Geometry check sheet. Reference: the model listing, model coordinates, mm. A direction names the side the tool comes from. Round coordinates to 2 decimals unless told otherwise and drop trailing zeros. Write each loop counter-clockwise with the first axis right and the second up, starting at its lowest first coordinate (ties: lowest second). Pieces come first, ordered by that corner, then holes.
from build123d import *

# Parameters (mm, degrees)
F0_W     = 10
F0_H     = 10
F1_DEPTH = 2
F2_W     = 2
F2_H     = 10
F3_DEPTH = 8
F5_DEPTH = 50


with BuildPart() as f1:
    # F0 (on Top) → F1 (new body)
    with BuildSketch(Plane.XY):
        Rectangle(F0_W, F0_H)
    extrude(amount=F1_DEPTH)

    # F2 (on face) → F3 (join)
    with BuildSketch(Plane.XY.offset(2)):
        with Locations((-4, 0)):
            Rectangle(F2_W, F2_H)
        with Locations((4, 0)):
            Rectangle(F2_W, F2_H)
    extrude(amount=F3_DEPTH)

    # F4 (on face) → F5 (join)
    with BuildSketch(Plane(origin=(0, 5, 0), x_dir=(-1, 0, 0), z_dir=(0, 1, 0))):
        Polygon((-3, 10), (-5, 10), (-5, 0), (5, 0), (5, 10), (3, 10), (3, 2), (-3, 2), align=None)
    extrude(amount=F5_DEPTH)


solid = f1.part
1. Section check B-B (y = 9). Record the cut outline in (x, z), plus the area to 3 significant figures.
2. Section check A-A (z = 6.25). Record the cut outline in (x, y).
3. Depth check by flat-ended pin: pin 1 Ø3 at (x, y) = (0, 33.5) entering from +Z. Enter the tip coordinate at first touch or a pass-through.
4. Access from +Z, -Z, +X, -X, +Y, -Y to the whole of each face (thin tool, end or side, straight path). Record for faces 1 (the face through (3, 25, 6)), 2 (the face through (-4, 25, 10)).
5. Section check C-C (x = 0.75). Record the cut outline in (y, z), plus the area to 3 significant figures.
6. Scan lines: line 1 along X through (y, z) = (39.5, 8.75); line 2 along Z through (x, y) = (1.75, 5). Record each from-to range of solid material in increasing order.
7. Release check for a two-part mould opening along Y. For faces 3 (the face through (0.1, 55, 1.7)), 4 (the face through (4, 25, 10)), 5 (the face through (-0.1, -5, 1.6)) record: +Y half, -Y half, draft (parallel to the pull), parting line (faces both ways), or undercut.
Results below:
1. outline: (-5, 0) - (5, 0) - (5, 10) - (3, 10) - (3, 2) - (-3, 2) - (-3, 10) - (-5, 10) - close
1. area: 52.0 mm2
2. outline: (-5, -5) - (-3, -5) - (-3, 55) - (-5, 55) - close; (3, -5) - (5, -5) - (5, 55) - (3, 55) - close
3. pin 1: stops at z = 2
4. face 1: +Z, +Y, -Y
4. face 2: +Z, +X, -X, +Y, -Y
5. outline: (-5, 0) - (55, 0) - (55, 2) - (-5, 2) - close
5. area: 120 mm2
6. line 1: x = -5 to -3, 3 to 5
6. line 2: z = 0 to 2
7. face 3: +Y half
7. face 4: draft
7. face 5: -Y half
